Read the model definition and answer for the solid it produces. Units are mm, in the model's axes. A direction names the side the tool comes from. Give positions to 0.01 mm unless a question says otherwise; leave off trailing zeros. Order: outer loops, then holes, each group sorted by start corner. A loop starts at its lowest first (then second) coordinate and runs counter-clockwise, first axis right, second up.
Item 1: The mould has two halves that part along X. Classify faces 5 (the face through (0.285, 34.699, 9.633)), 6 (the face through (17.94, 18.9, 3.45)), 7 (the face through (8, 25, 14)): +X half, -X half, draft (parallel to the pull), parting line (faces both ways), or undercut.
Item 2: Which of the six approach directions +Z, -Z, +X, -X, +Y, -Y give full straight-line access (tool end or side, diameter ignored) to faces 1 (the face through (7, 25, 16)), 2 (the face through (4.78, 4.77, 12.1)), 3 (the face through (4.15, 8, 12)), 4 (the face through (7, 14.5, 14))?
Item 3: A cutting plane is placed at B-B (z = 14). Write down the section's boundary in (x, y), plus the area to 3 significant figures.
Item 4: A cutting plane is placed at A-A (z = 6). Write down the section's boundary in (x, y), plus the area to 3 significant figures.
Item 5: Given pin 1 Ø5 at (x, z) = (14, 15) entering from +Y; pin 2 Ø3 at (y, z) = (20, 14.5) entering from +X; pin 3 Ø11 at (x, z) = (11, 15) entering from +Y; pin 4 Ø5.5 at (x, y) = (12.51, 20.4) entering from -Z, each flat-ended and moving along its own axis, determine where each tip first touches the part or whether it passes through.
Item 6: Find the intervals of material crossed by line 1 along Y through (x, z) = (22.5, 12.25); line 2 along X through (y, z) = (20, 15.25); line 3 along Z through (x, y) = (16, 14.5), in increasing order.
Item 7: A cutting plane is placed at C-C (y = 12). Write down the section's boundary in (x, z).
Item 8: A cutting plane is placed at D-D (x = 23.5). Write down the section's boundary in (y, z), plus the area to 3 significant figures.
from build123d import *

# Parameters (mm, degrees)
F1_DEPTH  = 19
F3_DEPTH  = 14
F4_R      = 3.5
F5_DEPTH  = 7
F6_DEPTH  = 7
F7_DEPTH  = 25
F8_DEPTH  = 14
F9_R      = 1
F2_W      = 2.5
F2_H      = 20.5
F10_DEPTH = 3


with BuildPart() as f1:
    # F0 (on Top) → F1 (new body)
    with BuildSketch(Plane.XY):
        Polygon((0, 35), (0, 0), (35, 0), (35, 8), (8, 35), align=None)
    extrude(amount=F1_DEPTH)

    # F2 (on face) → F3 (cut)
    with BuildSketch(Plane.XY.offset(19)):
        Polygon((2.5, 2.5), (35, 2.5), (35, 4.15), (5.4, 4.15), (4.15, 5.4), (4.15, 11.4), (5.5, 11.4), (5.5, 13.5), (5.5, 14.5), (5.5, 35), (2.5, 35), align=None)
    extrude(amount=-F3_DEPTH, mode=Mode.SUBTRACT)

    # F4 (on face) → F5 (cut)
    with BuildSketch(Plane.XY):
        Polygon((18.7922096033, 22.0864700531), (14.1960155256, 26.6826641308), (7.9174976548, 25.0003403376), (6.2351738616, 18.7218224668), (10.8313679393, 14.125628389), (17.1098858102, 15.8079521822), align=None)
        with Locations((12.5136917325, 20.4041462599)):
            Circle(F4_R, mode=Mode.SUBTRACT)
    extrude(amount=F5_DEPTH, mode=Mode.SUBTRACT)

    # F2 (on face) → F6 (cut)
    with BuildSketch(Plane.XY.offset(19)):
        Polygon((8, 14.5), (5.5, 14.5), (5.5, 13.5), (29.5, 13.5), (8, 35), align=None)
    extrude(amount=-F6_DEPTH, mode=Mode.SUBTRACT)

    # F4 (on face) → F7 (cut)
    with BuildSketch(Plane.XY):
        with Locations((12.5136917325, 20.4041462599)):
            Circle(F4_R)
    extrude(amount=F7_DEPTH, mode=Mode.SUBTRACT)

    # F2 (on face) → F8 (cut)
    with BuildSketch(Plane.XY.offset(19)):
        Polygon((2.5, 2.5), (35, 2.5), (35, 4.15), (5.4, 4.15), (4.15, 5.4), (4.15, 11.4), (5.5, 11.4), (5.5, 13.5), (5.5, 14.5), (5.5, 35), (2.5, 35), align=None)
        Polygon((5.5, 11.4), (31.6, 11.4), (29.5, 13.5), (5.5, 13.5), align=None)
    extrude(amount=-F8_DEPTH, mode=Mode.SUBTRACT)

    # F9
    f9_edges = [f1.edges().sort_by_distance(p)[0] for p in [
        (0, 35, 9.5),
        (0, 0, 9.5),
        (0, 17.5, 0),
        (0, 17.5, 19),
        (35, 0, 9.5),
        (17.5, 0, 0),
        (17.5, 0, 19),
    ]]
    fillet(f9_edges, radius=F9_R)

    # F2 (on face) → F10 (cut)
    with BuildSketch(Plane.XY.offset(19)):
        with Locations((6.75, 24.75)):
            Rectangle(F2_W, F2_H)
    extrude(amount=-F10_DEPTH, mode=Mode.SUBTRACT)


solid = f1.part
Response values:
1. face 5: -X half
1. face 6: undercut
1. face 7: +X half
2. face 1: +Z, +X, +Y
2. face 2: +Z
2. face 3: +Z, +Y
2. face 4: +Z, +X
3. outline: (0, 1) arc R1 ccw to (1, 0) - (34, 0) arc R1 ccw to (35, 1) - (35, 2.5) - (2.5, 2.5) - (2.5, 35) - (1, 35) arc R1 ccw to (0, 34) - close; (4.15, 5.4) - (5.4, 4.15) - (35, 4.15) - (35, 8) - (31.6, 11.4) - (4.15, 11.4) - close; (5.5, 14.5) - (8, 14.5) - (8, 35) - (5.5, 35) - close
3. area: 436 mm2
4. outline: (0, 1) arc R1 ccw to (1, 0) - (34, 0) arc R1 ccw to (35, 1) - (35, 2.5) - (2.5, 2.5) - (2.5, 35) - (1, 35) arc R1 ccw to (0, 34) - close; (4.15, 5.4) - (5.4, 4.15) - (35, 4.15) - (35, 8) - (31.6, 11.4) - (4.15, 11.4) - close; (5.5, 13.5) - (29.5, 13.5) - (8, 35) - (5.5, 35) - close; hole (6.24, 18.72) - (10.83, 14.13) - (17.11, 15.81) - (18.79, 22.09) - (14.2, 26.68) - (7.92, 25) - close
4. area: 560 mm2
5. pin 1: stops at y = 11.4
5. pin 2: stops at x = 8
5. pin 3: stops at y = 35
5. pin 4: passes through
6. line 1: y = 0 to 2.5, 4.15 to 11.4
6. line 2: x = 0 to 2.5, 5.5 to 8
6. line 3: z = 0 to 12
7. outline: (0, 1) arc R1 ccw to (1, 0) - (31, 0) - (31, 5) - (2.5, 5) - (2.5, 19) - (1, 19) arc R1 ccw to (0, 18) - close
8. outline: (0, 1) arc R1 ccw to (1, 0) - (19.5, 0) - (19.5, 12) - (13.5, 12) - (13.5, 5) - (11.4, 5) - (11.4, 19) - (4.15, 19) - (4.15, 5) - (2.5, 5) - (2.5, 19) - (1, 19) arc R1 ccw to (0, 18) - close
8. area: 276 mm2
